Source: CAD feature listing. Evaluate the final solid. Frame: model axes, mm. A direction names the side the tool comes from. Coordinates: 2 decimals unless noted, no trailing zeros. Order: outer loops, then holes, each group sorted by start corner. A loop starts at its lowest first (then second) coordinate and runs counter-clockwise, first axis right, second up. Notation, with made-up numbers: (-1, 26) -> (7, 26) arc R26 cw to (7, 62) -> close; hole circle Ø11 at (-12, 43.5). An arc over 180 degrees is marked (long way). Write item = value, one per line. Start each with the question number.
Item 1: Section query A-A (x = -11). Output: boundary loops of the cut face in (y, z), then the cut area to 3 significant figures.
Item 2: Set-up query: faces 4 (the cylindrical face through (-12.387, 5.252, 3.944)), 5 (the flat face through (0, 2, 8)). Return all of +Z, -Z, +X, -X, +Y, -Y with unobstructed straight access to the full face (end or side cutting, diameter ignored); none if empty.
Item 3: Ray query, line 1 along X through (y, z) = (12, 7.25); line 2 along Y through (x, z) = (-11, 6.5); line 3 along Z through (x, y) = (5.5, -4). Return the intervals inside material, ascending. Write a range as [from, to].
Item 4: Section query D-D (x = 8.5). Output: boundary loops of the cut face in (y, z), then the cut area to 3 significant figures.
Item 5: Mould query, pull axis Y, two halves, no side actions, for faces 1 (the cylindrical face through (9.613, 5.252, 3.944)), 2 (the flat face through (0, -20, 28)), 3 (the flat face through (0, 21.5, 4)). Classes: released by +Y, released by -Y, zero draft, split by the parting line, or undercut.
Item 6: Section query B-B (y = 11.5). Output: boundary loops of the cut face in (x, z), then the cut area to 3 significant figures.
Item 7: Section query C-C (z = 5.5). Output: boundary loops of the cut face in (x, y).
Item 8: Contact query for flat-ended pins moving along their axis: pin 1 (3 mm diameter, centred on x = -15, y = -5, fed in from +Z); pin 2 (5 mm diameter, centred on x = -15, z = 15, fed in from +Y). Output: stop coordinate, or through.
```python
from build123d import *

# Parameters (mm, degrees)
CROQUIS7_W              = 44.8
CROQUIS7_H              = 43
CROQUIS7_R              = 6.4
SALIENTE_EXTRUIR4_DEPTH = 8
CROQUIS8_W              = 44.8
CROQUIS8_H              = 3
SALIENTE_EXTRUIR5_DEPTH = 20


with BuildPart() as part:
    # Croquis7 → Saliente-Extruir4 (new body)
    with BuildSketch(Plane.XY):
        Rectangle(CROQUIS7_W, CROQUIS7_H)
        with Locations((-11, 11.5)):
            Circle(CROQUIS7_R, mode=Mode.SUBTRACT)
        with Locations((11, 11.5)):
            Circle(CROQUIS7_R, mode=Mode.SUBTRACT)
    extrude(amount=SALIENTE_EXTRUIR4_DEPTH)

    # Croquis8 → Saliente-Extruir5 (add)
    with BuildSketch(Plane.XY.offset(8)):
        with Locations((0, -20)):
            Rectangle(CROQUIS8_W, CROQUIS8_H)
    extrude(amount=SALIENTE_EXTRUIR5_DEPTH)


solid = part.part
```
Computed:
q1.outline = (-21.5, 0) -> (5.1, 0) -> (5.1, 8) -> (-18.5, 8) -> (-18.5, 28) -> (-21.5, 28) -> close; (17.9, 0) -> (21.5, 0) -> (21.5, 8) -> (17.9, 8) -> close
q1.area = 302 mm^2
q2.face_4 = +Z, -Z
q2.face_5 = +Z, +X, -X, +Y
q3.line_1 = [-22.4, -17.38], [-4.62, 4.62], [17.38, 22.4]
q3.line_2 = [-21.5, 5.1], [17.9, 21.5]
q3.line_3 = [0, 8]
q4.outline = (-21.5, 0) -> (5.61, 0) -> (5.61, 8) -> (-18.5, 8) -> (-18.5, 28) -> (-21.5, 28) -> close; (17.39, 0) -> (21.5, 0) -> (21.5, 8) -> (17.39, 8) -> close
q4.area = 310 mm^2
q5.face_1 = undercut
q5.face_2 = zero draft
q5.face_3 = released by +Y
q6.outline = (-22.4, 0) -> (-17.4, 0) -> (-17.4, 8) -> (-22.4, 8) -> close; (-4.6, 0) -> (4.6, 0) -> (4.6, 8) -> (-4.6, 8) -> close; (17.4, 0) -> (22.4, 0) -> (22.4, 8) -> (17.4, 8) -> close
q6.area = 154 mm^2
q7.outline = (-22.4, -21.5) -> (22.4, -21.5) -> (22.4, 21.5) -> (-22.4, 21.5) -> close; hole circle Ø12.8 at (-11, 11.5); hole circle Ø12.8 at (11, 11.5)
q8.pin_1 = 8
q8.pin_2 = -18.5
